Check sheet for the modelled part. Datum: model origin and axes. Units: mm. Round coordinates to 2 decimals unless told otherwise and drop trailing zeros. Loops run counter-clockwise (first coordinate to the right, second up) from the corner with the lowest first, then second, coordinate; pieces in that order, holes last. Notation, with made-up numbers: M 17,9.5 L 28,9.5 A17 ccw 28,18.5 Z; hole C 47.25,84.5 d4. An arc over 180 degrees is marked long. Write item = value, one per line. Start each with the question number.
(1) Scan lines: L1, parallel to X at y = 0.6, z = 39; L2, parallel to X at y = 0.15, z = 38.5; L3, parallel to Z at x = 1, y = 0.25. Record each from-to range of solid material in increasing order. Write a range as from..to.
(2) Cross-section at C-C on z = 49. Record the boundary of the cut face in (x, y), plus the area to 3 significant figures.
(3) Cross-section at B-B on x = 0. Record the boundary of the cut face in (y, z), plus the area to 3 significant figures.
(4) Go/stop test with a flat-tipped pin: P1, Ø1.9, axis at x = -27.75, z = 38.03, coming from the -Y side. Record where the tip stops, or that it passes through.
(5) Cross-section at A-A on y = 0.2. Record the boundary of the cut face in (x, z).
(6) Mould release check, pull along X, two halves, no side actions. Record for faces 1 (the face through (-0.47, 0.39, -39.47)), 2 (the face through (0, 0, 10)), 3 (the face through (0.704, 0.394, 70.024)): pulls with the +X half, pulls with the -X half, needs draft (parallel to the pull), parting line crosses it, or undercut.
from build123d import *

# Parameters (mm, degrees)
BOSS_EXTRUDE1_DEPTH = 0.8
SKETCH2_R           = 1.6
CUT_EXTRUDE1_DEPTH  = 78.000105196


with BuildPart() as part:
    # Sketch1 → Boss-Extrude1 (new body)
    with BuildSketch(Plane(origin=(0, 0, 0), x_dir=(1, 0, 0), z_dir=(0, 1, 0))):
        with BuildLine():
            Line((-32, -38.031251597), (-32, 48.282157899))
            ThreePointArc((-32, 48.282157899), (0, 39.468748403), (32, 48.282157899))
            Line((32, 48.282157899), (32, -38.031251597))
            ThreePointArc((32, -38.031251597), (0, -70.031251597), (-32, -38.031251597))
        make_face()
    extrude(amount=BOSS_EXTRUDE1_DEPTH)

    # Sketch2 → Cut-Extrude1 (cut, through all)
    with BuildSketch(Plane.XZ):
        with Locations(Location((27.75, 38.031251597, 0), (0, 0, 270))):
            Circle(SKETCH2_R)
        with Locations(Location((-27.75, 38.031251597, 0), (0, 0, 270))):
            Circle(SKETCH2_R)
        with Locations(Location((27, -38.282157899, 0), (0, 0, 270))):
            Circle(SKETCH2_R)
        with Locations(Location((-27, -38.282157899, 0), (0, 0, 270))):
            Circle(SKETCH2_R)
    extrude(amount=-CUT_EXTRUDE1_DEPTH, mode=Mode.SUBTRACT)


solid = part.part
Result:
q1.L1 = -31.99..-29.02, -26.48..26.48, 29.02..31.99
q1.L2 = -32..-29.28, -26.22..26.22, 29.28..32
q1.L3 = -39.48..70.02
q2.outline = M -30.06,0 L 30.06,0 L 30.06,0.8 L -30.06,0.8 Z
q2.area = 48.1 mm^2
q3.outline = M 0,-39.47 L 0.8,-39.47 L 0.8,70.03 L 0,70.03 Z
q3.area = 87.6 mm^2
q4.P1 = through
q5.outline = M -32,-48.28 A62.5 cw 32,-48.28 L 32,38.03 A32 ccw -32,38.03 Z; hole C -27.75,38.03 d3.2; hole C -27,-38.28 d3.2; hole C 27,-38.28 d3.2; hole C 27.75,38.03 d3.2
q6.face_1 = undercut
q6.face_2 = needs draft
q6.face_3 = parting line crosses it
